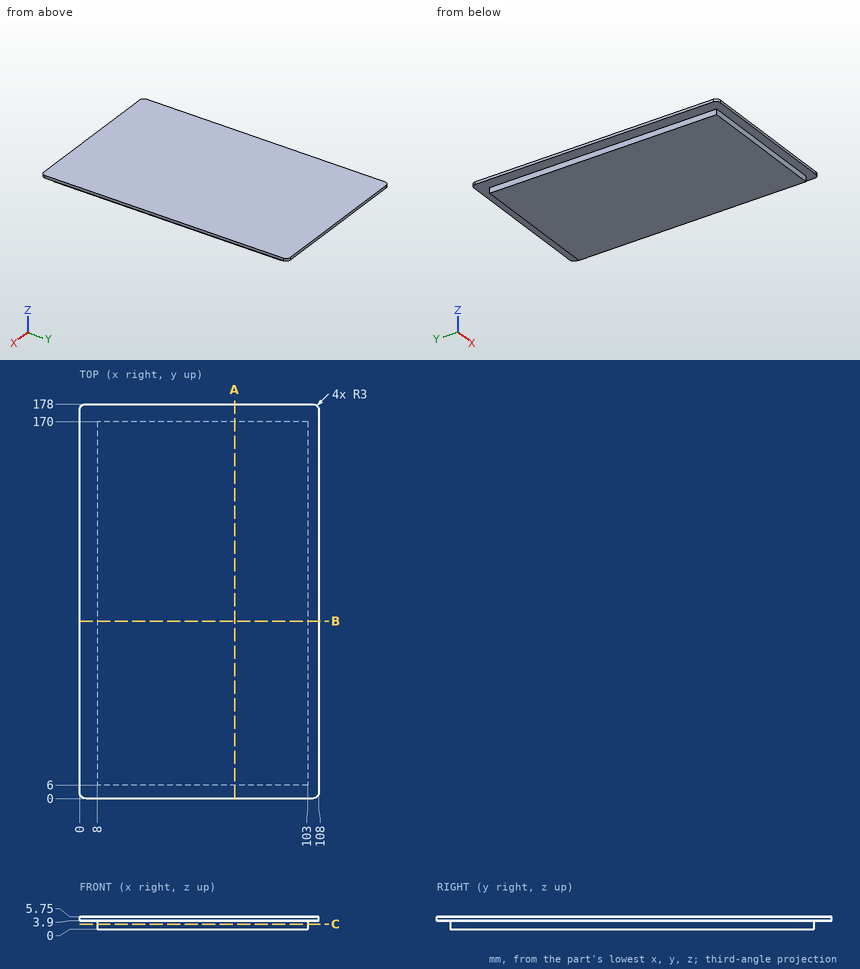
Print and shaded views of the part. All mm, measured from the part's lowest x, y and z. Coordinates: 2 decimals unless noted, no trailing zeros. Loops run counter-clockwise (first coordinate to the right, second up) from the corner with the lowest first, then second, coordinate; pieces in that order, holes last. Notation, with made-up numbers: (10, -18.75) - (65, -18.75) arc R23 ccw to (65, 19.25) - close; hole circle Ø10 at (84, 68). An arc over 180 degrees is marked (long way). Write item = value, one per line. Start each with the question number.
Item 1: Drop flat-ended pins along their axis: pin 1 Ø3 at (x, z) = (72, 1.5) entering from +Y; pin 2 Ø1.2 at (x, z) = (48, 1.5) entering from -Y; pin 3 Ø2 at (y, z) = (79, 1) entering from -X. Give the stop position or say it passes through.
Item 2: Saw through at B-B, the plane y = 80. List the corners of the cut face in (x, z), then the cut area to 3 significant figures.
Item 3: Wall check: probe 1 along X at (y, z) = (20, 1.6); probe 2 along Y at (x, z) = (72, 1.9). Give the ranges that are in metal, low to high. Write a range as [from, to].
Item 4: Saw through at A-A, the plane x = 70. List the corners of the cut face in (y, z), then the cut area to 3 significant figures.
Item 5: Saw through at C-C, the plane z = 2.35. List the corners of the cut face in (x, y), then the cut area to 3 significant figures.
Answers:
q1.pin_1 = 170
q1.pin_2 = 6
q1.pin_3 = 8
q2.outline = (0, 3.9) - (8, 3.9) - (8, 0) - (103, 0) - (103, 3.9) - (108, 3.9) - (108, 5.75) - (0, 5.75) - close
q2.area = 570 mm2
q3.probe_1 = [8, 103]
q3.probe_2 = [6, 170]
q4.outline = (0, 3.9) - (6, 3.9) - (6, 0) - (170, 0) - (170, 3.9) - (178, 3.9) - (178, 5.75) - (0, 5.75) - close
q4.area = 969 mm2
q5.outline = (8, 6) - (103, 6) - (103, 170) - (8, 170) - close
q5.area = 15,600 mm2
